Verification items for this drawing (mm, ordinates from the low corner). A direction names the side the tool comes from. Coordinates: 2 decimals unless noted, no trailing zeros. Loops run counter-clockwise (first coordinate to the right, second up) from the corner with the lowest first, then second, coordinate; pieces in that order, holes last. Notation, with made-up numbers: M 24.5,37 L 77.5,37 A12 cw 77.5,52 Z; hole C 70.25,25 d8. An arc over 180 degrees is marked long. Use CSV: the item, a comma, the result in double quotes.
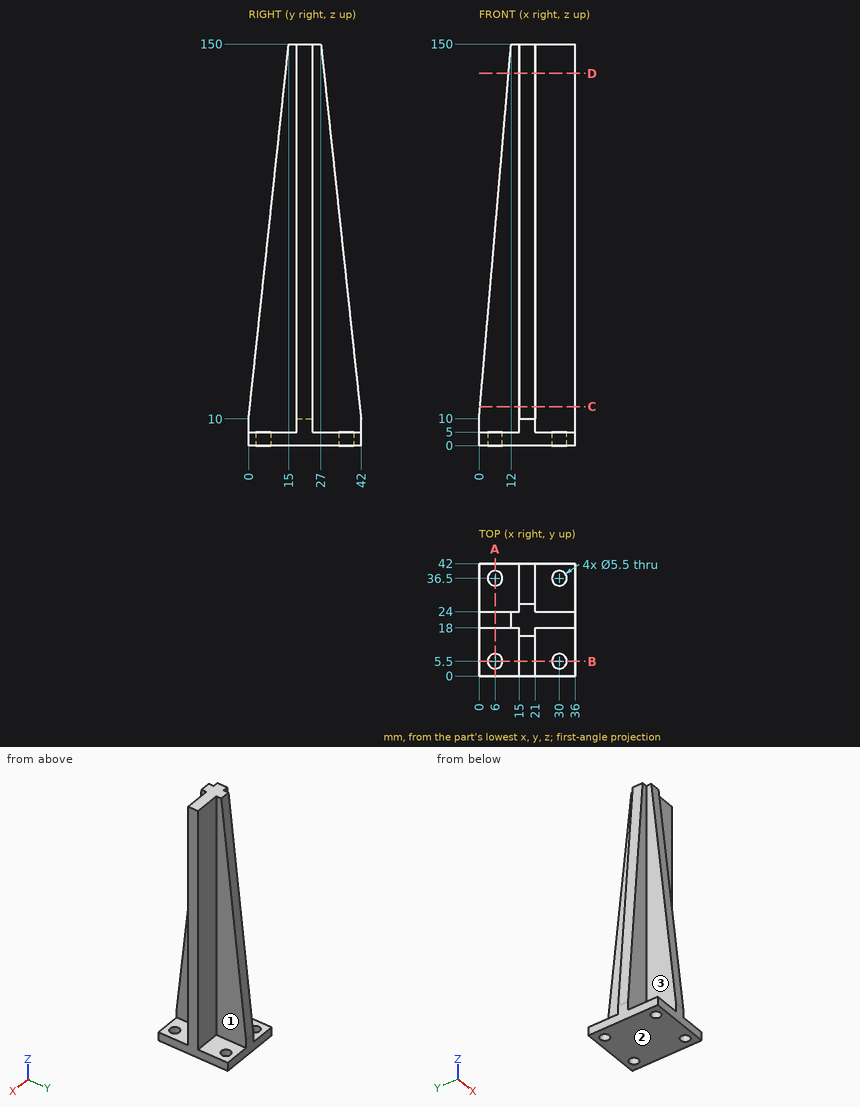
1. Section check A-A, the plane x = 6. Record the cut outline in (y, z), plus the area to 3 significant figures.
The answers:
outline,"M 0,0 L 2.75,0 L 2.75,5 L 0,5 Z; M 8.25,0 L 33.75,0 L 33.75,5 L 24,5 L 24,80 L 18,80 L 18,5 L 8.25,5 Z; M 39.25,0 L 42,0 L 42,5 L 39.25,5 Z"
area,"605 mm^2"
2. Section check C-C, the plane z = 14.5. Record the cut outline in (x, y).
The answers:
outline,"M 0.39,18 L 15,18 L 15,0.48 L 21,0.48 L 21,18 L 36,18 L 36,24 L 21,24 L 21,41.52 L 15,41.52 L 15,24 L 0.39,24 Z"
3. Section check B-B, the plane y = 5.5. Record the cut outline in (x, z), plus the area to 3 significant figures.
The answers:
outline,"M 0,0 L 3.25,0 L 3.25,5 L 0,5 Z; M 8.75,0 L 27.25,0 L 27.25,5 L 21,5 L 21,61.33 L 15,61.33 L 15,5 L 8.75,5 Z; M 32.75,0 L 36,0 L 36,5 L 32.75,5 Z"
area,"463 mm^2"
4. Section check D-D, the plane z = 139. Record the cut outline in (x, y), plus the area to 3 significant figures.
The answers:
outline,"M 11.06,18 L 15,18 L 15,13.82 L 21,13.82 L 21,18 L 36,18 L 36,24 L 21,24 L 21,28.18 L 15,28.18 L 15,24 L 11.06,24 Z"
area,"200 mm^2"
5. Gauge pin test, flat ends, axial feed: P1, Ø9, axis at y = 37, z = 88.5, coming from the +X side; P2, Ø8, axis at x = 14, z = 35.5, coming from the -Y side; P3, Ø4.5, axis at x = 7, y = 30.5, coming from the +Z side; P4, Ø5, axis at x = 30, y = 36.5, coming from the +Z side. Record the tip position at first contact, or that the pin passes through.
The answers:
P1,"x = 21"
P2,"y = 2.32"
P3,"z = 5"
P4,"through"
6. Set-up check for the marked faces 1, 2 and 3: record each of +Z, -Z, +X, -X, +Y, -Y from which the full face is reachable in a straight line by a thin tool's end or side.
The answers:
face 1,"+Z, +X, +Y"
face 2,"-Z, +X, -X, +Y, -Y"
face 3,"+Z, -X, -Y"
7. Thickness scan on line 1 (Y direction, x = 6, z = 4); line 2 (X direction, y = 5, z = 1); line 3 (Y direction, x = 32, z = 116.5). Record the ranges inside material, lowest first. Write a range as [from, to].
The answers:
line 1,"[0, 2.75], [8.25, 33.75], [39.25, 42]"
line 2,"[0, 3.3], [8.7, 27.3], [32.7, 36]"
line 3,"[18, 24]"
